from build123d import *

# Parameters (mm, degrees)
SKETCH1_W           = 126
SKETCH1_H           = 126
BOSS_EXTRUDE1_DEPTH = 5
SKETCH3_R           = 12.5
BOSS_EXTRUDE2_DEPTH = 7.5
SKETCH4_R           = 2.95
CUT_EXTRUDE1_DEPTH  = 11.5
SKETCH6_R           = 2.5
CUT_EXTRUDE2_DEPTH  = 179.628805068
CHAMFER1_SIZE       = 10
CHAMFER1_SIZE_2     = 7.26542528
SKETCH9_W           = 5
SKETCH9_H           = 75
BOSS_EXTRUDE4_DEPTH = 3
SKETCH10_W          = 3
SKETCH10_H          = 3
CUT_EXTRUDE4_DEPTH  = 179.370401132
SKETCH11_W          = 5
SKETCH11_H          = 108
BOSS_EXTRUDE5_DEPTH = 3
SKETCH12_W          = 3
SKETCH12_H          = 3
CUT_EXTRUDE5_DEPTH  = 179.370401132


with BuildPart() as part:
    # Sketch1 → Boss-Extrude1 (new body)
    with BuildSketch(Plane(origin=(0, 0, 0), x_dir=(1, 0, 0), z_dir=(0, 1, 0))):
        with Locations((63, 63)):
            Rectangle(SKETCH1_W, SKETCH1_H)
    extrude(amount=BOSS_EXTRUDE1_DEPTH)

    # Sketch3 → Boss-Extrude2 (add)
    with BuildSketch(Plane(origin=(0, 5, 0), x_dir=(1, 0, 0), z_dir=(0, 1, 0))):
        with Locations(Location((108.6, 108.6, 0), (0, 0, 90))):
            Circle(SKETCH3_R)
    extrude(amount=BOSS_EXTRUDE2_DEPTH)

    # Sketch4 → Cut-Extrude1 (cut)
    with BuildSketch(Plane.XZ):
        with Locations(Location((108.6, -108.6, 0), (0, 0, 270))):
            Circle(SKETCH4_R)
    extrude(amount=-CUT_EXTRUDE1_DEPTH, mode=Mode.SUBTRACT)

    # Sketch6 → Cut-Extrude2 (cut, through all)
    with BuildSketch(Plane(origin=(0, 12.5, 0), x_dir=(1, 0, 0), z_dir=(0, 1, 0))):
        with Locations(Location((108.6, 108.6, 0), (0, 0, 270))):
            Circle(SKETCH6_R)
    extrude(amount=-CUT_EXTRUDE2_DEPTH, mode=Mode.SUBTRACT)

    # Chamfer1
    # the kernel refuses this chamfer: 10, 7.26542528 mm, written as the material it takes off along each edge
    with BuildSketch(Plane(origin=(108.6, 12.5, -108.6), x_dir=(0, 0, -1), z_dir=(1, 0, 0))) as chamfer1_piece_1_section:
        Polygon((12.5, -CHAMFER1_SIZE), (12.5 - CHAMFER1_SIZE_2, 0), (12.5, 0), align=None)
    chamfer1_piece_1 = revolve(axis=Axis((108.6, 12.5, -108.6), (0, 1, 0)), mode=Mode.PRIVATE)
    chamfer1_piece_1 = split(chamfer1_piece_1, bisect_by=Plane(origin=(108.6, 5, -100.650989912), z_dir=(0, 1, 0)), keep=Keep.TOP, mode=Mode.PRIVATE)
    add(chamfer1_piece_1, mode=Mode.SUBTRACT)

    # Sketch9 → Boss-Extrude4 (add)
    with BuildSketch(Plane(origin=(0, 5, 0), x_dir=(1, 0, 0), z_dir=(0, 1, 0))):
        with Locations((108.6, 48.95817816)):
            Rectangle(SKETCH9_W, SKETCH9_H)
    extrude(amount=BOSS_EXTRUDE4_DEPTH)

    # Sketch10 → Cut-Extrude4 (cut, through all)
    with BuildSketch(Plane(origin=(0, 8, 0), x_dir=(1, 0, 0), z_dir=(0, 1, 0))):
        with Locations((108.6, 83.95817816)):
            Rectangle(SKETCH10_W, SKETCH10_H)
        with Locations((108.6, 69.958932274)):
            Rectangle(SKETCH10_W, SKETCH10_H)
        with Locations((108.6, 55.959686388)):
            Rectangle(SKETCH10_W, SKETCH10_H)
        with Locations((108.6, 41.960440502)):
            Rectangle(SKETCH10_W, SKETCH10_H)
        with Locations((108.6, 27.961194616)):
            Rectangle(SKETCH10_W, SKETCH10_H)
        with Locations((108.6, 13.96194873)):
            Rectangle(SKETCH10_W, SKETCH10_H)
    extrude(amount=-CUT_EXTRUDE4_DEPTH, mode=Mode.SUBTRACT)

    # Sketch11 → Boss-Extrude5 (add)
    with BuildSketch(Plane(origin=(0, 5, 0), x_dir=(1, 0, 0), z_dir=(0, 1, 0))):
        with Locations((8.881061813, 63)):
            Rectangle(SKETCH11_W, SKETCH11_H)
    extrude(amount=BOSS_EXTRUDE5_DEPTH)

    # Sketch12 → Cut-Extrude5 (cut, through all)
    with BuildSketch(Plane(origin=(0, 8, 0), x_dir=(1, 0, 0), z_dir=(0, 1, 0))):
        with Locations((8.881061813, 114.5)):
            Rectangle(SKETCH12_W, SKETCH12_H)
        with Locations((8.881061813, 93.900163021)):
            Rectangle(SKETCH12_W, SKETCH12_H)
        with Locations((8.881061813, 73.300326041)):
            Rectangle(SKETCH12_W, SKETCH12_H)
        with Locations((8.881061813, 52.700489062)):
            Rectangle(SKETCH12_W, SKETCH12_H)
        with Locations((8.881061813, 32.100652082)):
            Rectangle(SKETCH12_W, SKETCH12_H)
        with Locations((8.881061813, 11.500815103)):
            Rectangle(SKETCH12_W, SKETCH12_H)
    extrude(amount=-CUT_EXTRUDE5_DEPTH, mode=Mode.SUBTRACT)


solid = part.part
The listing builds one solid part. Answer for the finished solid, in the listing's coordinates (mm). A direction names the side the tool comes from. Give positions to 0.01 mm unless a question says otherwise; leave off trailing zeros. Write each loop counter-clockwise with the first axis right and the second up, starting at its lowest first coordinate (ties: lowest second). Pieces come first, ordered by that corner, then holes.
1) For a pull along Z with two mould halves and no side action, classify faces 1 (the face through (109, 4, -29.461)), 2 (the face through (62, 0, -64)), 3 (the face through (109, 4, -40.46)), 4 (the face through (62, 2, 0)) as pulls with the +Z half, pulls with the -Z half, needs draft (parallel to the pull), parting line crosses it, or undercut.
2) Section C-C (y = 6.5) is taken. Count the separate pieces of the cut face and the enclosed holes in it, and give its area (3 significant figures).
3) A tool of negligible diameter and unlimited length cuts with its end or side. For faces 5 (the face through (109, 6, -86.458)), 6 (the face through (110.1, 4, -56)), 7 (the face through (108, 11.5, -106)), from which of +Z, -Z, +X, -X, +Y, -Y can it reach the whole face along a straight path? Write none if from no direction.
4) Find the intervals of material crossed by L1, parallel to X at y = 7, z = -108.6; L2, parallel to X at y = 7.75, z = -10.5; L3, parallel to Y at x = 69, z = -59, in increasing order.
5) Section A-A (z = -108.6) is taken. Write down the section's boundary in (x, y), and give its area (3 significant figures).
6) Given P1, Ø5, axis at y = 8.5, z = -13, coming from the +X side; P2, Ø1.5, axis at x = 72, y = 6.5, coming from the +Z side; P3, Ø3.5, axis at x = 108.5, y = 6.5, coming from the +Z side; P4, Ø3, axis at x = 110, z = -108.5, coming from the -Y side, each flat-ended and moving along its own axis, determine where each tip first touches the part or whether it passes through.
7) Section B-B (z = -66.5) is taken. Write down the section's boundary in (x, y).
Response:
1. face 1: undercut
1. face 2: needs draft
1. face 3: undercut
1. face 4: pulls with the +Z half
2. separate pieces: 3
2. enclosed holes: 13
2. area: 1,070 mm2
3. face 5: +X, +Y
3. face 6: +Y, -Y
3. face 7: -Y
4. L1: x = 6.38 to 11.38, 99.37 to 105.65, 111.55 to 117.83
4. L2: x = 6.38 to 7.38, 10.38 to 11.38
4. L3: y = 0 to 5
5. outline: (0, 0) - (105.65, 0) - (105.65, 11.5) - (106.1, 11.5) - (106.1, 12.5) - (103.37, 12.5) - (97.92, 5) - (11.38, 5) - (11.38, 8) - (6.38, 8) - (6.38, 5) - (0, 5) - close; (111.1, 11.5) - (111.55, 11.5) - (111.55, 0) - (126, 0) - (126, 5) - (119.28, 5) - (113.83, 12.5) - (111.1, 12.5) - close
5. area: 692 mm2
6. P1: stops at x = 111.1
6. P2: passes through
6. P3: stops at z = 0
6. P4: stops at y = 11.5
7. outline: (0, 0) - (126, 0) - (126, 5) - (111.1, 5) - (111.1, 8) - (106.1, 8) - (106.1, 5) - (11.38, 5) - (11.38, 8) - (6.38, 8) - (6.38, 5) - (0, 5) - close
